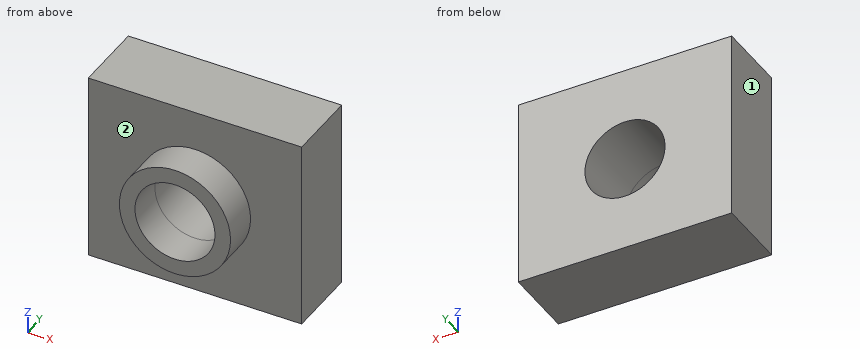
```python
from build123d import *

# Parameters (mm, degrees)
F0_W     = 75.245142
F0_H     = 67.105166
F1_DEPTH = 25.4
F2_R     = 14.122943
F3_DEPTH = 25.401
F2_R_2   = 19.605115
F4_DEPTH = 12.7


with BuildPart() as f1:
    # F0 (on Front) → F1 (new body)
    with BuildSketch(Plane.XZ):
        Rectangle(F0_W, F0_H)
    extrude(amount=F1_DEPTH)

    # F2 (on face) → F3 (cut, through all)
    with BuildSketch(Plane.XZ.offset(25.4)):
        Circle(F2_R)
    extrude(amount=-F3_DEPTH, mode=Mode.SUBTRACT)

    # F2 (on face) → F4 (join)
    with BuildSketch(Plane.XZ.offset(25.4)):
        Circle(F2_R_2)
        Circle(F2_R, mode=Mode.SUBTRACT)
    extrude(amount=F4_DEPTH)


solid = f1.part
```
Can you work these out from the model? Positions are in its coordinate system, mm. Face numbers are marked on the shaded views. A direction names the side the tool comes from. Round coordinates to 2 decimals unless told otherwise and drop trailing zeros. Loops run counter-clockwise (first coordinate to the right, second up) from the corner with the lowest first, then second, coordinate; pieces in that order, holes last.
Item 1: Please list where these lines run through material, in increasing order: L1, parallel to Z at x = 0, y = -13.25; L2, parallel to Z at x = 0, y = -28.5; L3, parallel to Y at x = -22.5, z = 5.
Item 2: Will these pins go through, and if not, where does the flat tip stop? pin 1 Ø1.5 at (x, z) = (-20.5, -1) entering from -Y; pin 2 Ø3 at (y, z) = (-28, 13.5) entering from +X.
Item 3: Suppose I cut it at B-B, the plane z = 0. Write out the boundary of the cut face in (x, y).
Item 4: Which directions (+Z, -Z, +X, -X, +Y, -Y) give clear straight access to the entire face, cutting with the end or side of a thin tool? Please do the marked faces 1 and 2.
Item 5: Suppose I cut it at A-A, the plane x = 0. Write out the boundary of the cut face in (y, z), then the cut area to 3 significant figures.
Item 6: Suppose I cut it at C-C, the plane y = -18.5. Write out the boundary of the cut face in (x, z), then the cut area to 3 significant figures.
Item 7: Suppose I cut it at D-D, the plane z = 15.5. Write out the boundary of the cut face in (x, y), then the cut area to 3 significant figures.
Reported:
1. L1: z = -33.55 to -14.12, 14.12 to 33.55
1. L2: z = -19.61 to -14.12, 14.12 to 19.61
1. L3: y = -25.4 to 0
2. pin 1: stops at y = -25.4
2. pin 2: stops at x = 15.5
3. outline: (-37.62, -25.4) - (-19.61, -25.4) - (-19.61, -38.1) - (-14.12, -38.1) - (-14.12, 0) - (-37.62, 0) - close; (14.12, -38.1) - (19.61, -38.1) - (19.61, -25.4) - (37.62, -25.4) - (37.62, 0) - (14.12, 0) - close
4. face 1: +Z, -Z, -X, +Y, -Y
4. face 2: -Y
5. outline: (-38.1, -19.61) - (-25.4, -19.61) - (-25.4, -33.55) - (0, -33.55) - (0, -14.12) - (-38.1, -14.12) - close; (-38.1, 14.12) - (0, 14.12) - (0, 33.55) - (-25.4, 33.55) - (-25.4, 19.61) - (-38.1, 19.61) - close
5. area: 1,130 mm2
6. outline: (-37.62, -33.55) - (37.62, -33.55) - (37.62, 33.55) - (-37.62, 33.55) - close; hole circle Ø28.25 at (0, 0)
6. area: 4,420 mm2
7. outline: (-37.62, -25.4) - (-12, -25.4) - (-12, -38.1) - (12, -38.1) - (12, -25.4) - (37.62, -25.4) - (37.62, 0) - (-37.62, 0) - close
7. area: 2,220 mm2
